from build123d import *

# Parameters (mm, degrees)
F0_W     = 184.15
F0_H     = 25.4
F0_R     = 5.207
F1_DEPTH = 31.369
F2_SIZE  = 1.5875
F3_SIZE  = 1.5875
F4_SIZE  = 1.5875


with BuildPart() as f1:
    # F0 (on Front) → F1 (new body)
    with BuildSketch(Plane.XZ):
        Rectangle(F0_W, F0_H)
        with Locations((-66.675, 0)):
            Circle(F0_R, mode=Mode.SUBTRACT)
        with Locations((-15.875, 0)):
            Circle(F0_R, mode=Mode.SUBTRACT)
        with Locations((34.925, 0)):
            Circle(F0_R, mode=Mode.SUBTRACT)
    extrude(amount=F1_DEPTH)

    # F2
    f2_edges = [f1.edges().sort_by_distance(p)[0] for p in [
        (92.075, -31.369, 0),
    ]]
    chamfer(f2_edges, length=F2_SIZE)

    # F3
    f3_edges = [f1.edges().sort_by_distance(p)[0] for p in [
        (-92.075, -31.369, 0),
    ]]
    chamfer(f3_edges, length=F3_SIZE)

    # F4
    f4_edges = [f1.edges().sort_by_distance(p)[0] for p in [
        (0, -31.369, 12.7),
        (0, -31.369, -12.7),
        (0, 0, -12.7),
        (0, 0, 12.7),
    ]]
    chamfer(f4_edges, length=F4_SIZE)


solid = f1.part
Geometry check sheet. Reference: the model listing, model coordinates, mm. Round coordinates to 2 decimals unless told otherwise and drop trailing zeros. Loops run counter-clockwise (first coordinate to the right, second up) from the corner with the lowest first, then second, coordinate; pieces in that order, holes last. Notation, with made-up numbers: (17, 49.25) - (61, 49.25) arc R29 cw to (61, 70.25) - close; hole circle Ø2 at (14.5, 73). An arc over 180 degrees is marked (long way). One line per question, with ' | ' between items. Start each with the question number.
1. Cross-section at B-B on y = -20.5. Record the cut outline in (x, z) (3 decimals), then the cut area to 3 significant figures.
2. Depth check by flat-ended pin: pin 1 (12 mm diameter, centred on x = 34.925, z = 0, fed in from +Y). Enter the tip coordinate at first touch or a pass-through.
3. Draft check along Z on faces 1 (the face through (-1, 0, 0)), 2 (the face through (-10.908, -15.465, 1.564)), 3 (the face through (-67.353, -15.465, 5.163)), 4 (the face through (-1, -15, -12.7)). Enter one of: released by +Z, released by -Z, zero draft, split by the parting line, or undercut.
4. Scan lines: line 1 (X direction, y = -20, z = 3.25) (3 decimals); line 2 (Z direction, x = -19, y = -26) (3 decimals); line 3 (X direction, y = -23, z = 3.5) (3 decimals). Record each from-to range of solid material in increasing order. Write a range as [from, to].
5. Cross-section at A-A on z = 0. Record the cut outline in (x, y) (1 decimal), then the cut area to 3 significant figures.
Taken from the geometry:
1) outline: (-92.075, -12.7) - (92.075, -12.7) - (92.075, 12.7) - (-92.075, 12.7) - close; hole circle Ø10.414 at (-66.675, 0); hole circle Ø10.414 at (-15.875, 0); hole circle Ø10.414 at (34.925, 0) | area: 4,420 mm²
2) pin 1: y = 0
3) face 1: zero draft | face 2: undercut | face 3: undercut | face 4: released by -Z
4) line 1: [-92.075, -70.743], [-62.607, -19.943], [-11.807, 30.857], [38.993, 92.075] | line 2: [-12.7, -4.165], [4.165, 12.7] | line 3: [-92.075, -70.53], [-62.82, -19.73], [-12.02, 31.07], [38.78, 92.075]
5) outline: (-92.1, -29.8) - (-90.5, -31.4) - (-71.9, -31.4) - (-71.9, 0) - (-92.1, 0) - close; (-61.5, -31.4) - (-21.1, -31.4) - (-21.1, 0) - (-61.5, 0) - close; (-10.7, -31.4) - (29.7, -31.4) - (29.7, 0) - (-10.7, 0) - close; (40.1, -31.4) - (90.5, -31.4) - (92.1, -29.8) - (92.1, 0) - (40.1, 0) - close | area: 4,790 mm²
